Build history of the part. All positions in model axes, mm. A direction names the side the tool comes from. Round coordinates to 2 decimals unless told otherwise and drop trailing zeros. Loops run counter-clockwise (first coordinate to the right, second up) from the corner with the lowest first, then second, coordinate; pieces in that order, holes last. Notation, with made-up numbers: (4.5, 69) - (61.5, 69) arc R4 cw to (61.5, 76) - close; hole circle Ø4 at (58.5, -6.5). An arc over 180 degrees is marked (long way). Use a Markdown table: item, result.
from build123d import *

# Parameters (mm, degrees)
SKETCH1_R           = 4
BOSS_EXTRUDE1_DEPTH = 2
SKETCH2_R           = 1
BOSS_EXTRUDE2_DEPTH = 18


with BuildPart() as part:
    # Sketch1 → Boss-Extrude1 (new body)
    with BuildSketch(Plane.XY):
        Circle(SKETCH1_R)
    extrude(amount=BOSS_EXTRUDE1_DEPTH)

    # Sketch2 → Boss-Extrude2 (add)
    with BuildSketch(Plane(origin=(0, 0, 0), x_dir=(-1, 0, 0), z_dir=(0, 0, -1))):
        Circle(SKETCH2_R)
    extrude(amount=BOSS_EXTRUDE2_DEPTH)

    # Sketch3 → Cut-Revolve1 (revolve, cut)
    with BuildSketch(Plane(origin=(0, 0, 0), x_dir=(0, 0, -1), z_dir=(1, 0, 0))):
        Polygon((-2, 4), (-1, 3), (0, 4), align=None)
    revolve(axis=Axis((0, 0, 3.115097116), (0, 0, -1)), mode=Mode.SUBTRACT)


solid = part.part
Q1. Cut at A-A, the plane y = 0. List the corners of the cut face in (x, z), plus the area to 3 significant figures.
Results found:
| item | result |
|---|---|
| outline | (-4, 0) - (-1, 0) - (-1, -18) - (1, -18) - (1, 0) - (4, 0) - (3, 1) - (4, 2) - (-4, 2) - (-3, 1) - close |
| area | 50.0 mm2 |
Q2. Which spindle directions (+Z, -Z, +X, -X, +Y, -Y) get a long thin tool onto all of the face, cutting with end or side? Do faces 1 (the face through (0, 0, 2)), 2 (the face through (0, -1, -9)). Say none if no direction does.
Results found:
| item | result |
|---|---|
| face 1 | +Z, +X, -X, +Y, -Y |
| face 2 | -Z |
Q3. Drop flat-ended pins along their axis: pin 1 (3 mm diameter, centred on x = 0, y = -3, fed in from -Z); pin 2 (4 mm diameter, centred on x = 1, z = -6.5, fed in from +Y). Give the stop position or say it passes through.
Results found:
| item | result |
|---|---|
| pin 1 | stops at z = 0 |
| pin 2 | stops at y = 1 |
Q4. Probe line 1 (Z direction, x = 0.75, y = -1); line 2 (Z direction, x = -3.25, y = 0.5); line 3 (X direction, y = 0.25, z = -6.75). List the from-to ranges inside material, lowest first.
Results found:
| item | result |
|---|---|
| line 1 | z = 0 to 2 |
| line 2 | z = 0 to 0.71, 1.29 to 2 |
| line 3 | x = -0.97 to 0.97 |
Q5. Cut at C-C, the plane z = -15.25. List the corners of the cut face in (x, y).
Results found:
| item | result |
|---|---|
| outline | circle Ø2 at (0, 0) |
